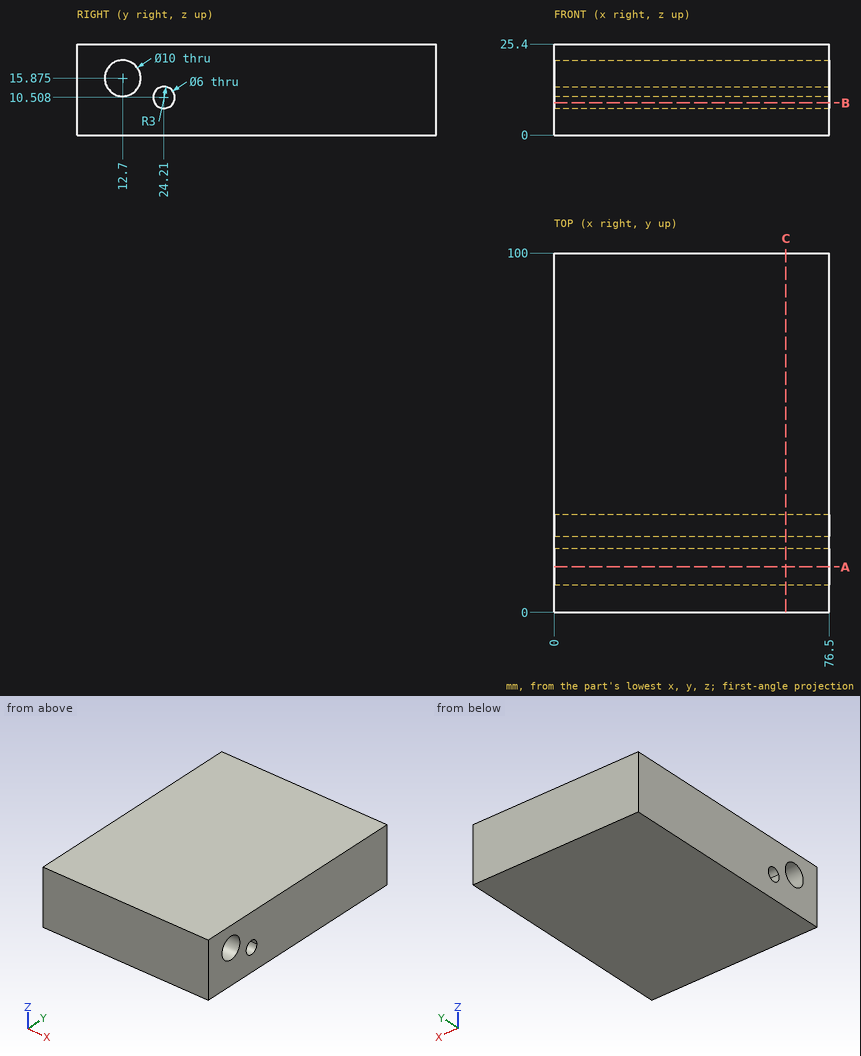
Design review of the part shown in the three views and the two pictorial views. Dimensions are in mm from the part's minimum x, y and z. Give positions to 0.01 mm unless a question says otherwise; leave off trailing zeros. Write each loop counter-clockwise with the first axis right and the second up, starting at its lowest first coordinate (ties: lowest second). Pieces come first, ordered by that corner, then holes.
Item 1: Insertion check: P1, Ø4, axis at x = 42, y = 51, coming from the -Z side. The pin has a flat end and moves straight along its axis. Give the tip position at first contact, or say it passes through.
Item 2: Take a section at C-C (x = 64.5). Give the boundary of the cut face in (y, z) (1 decimal), and give its area (3 significant figures).
Item 3: Take a section at A-A (y = 12.7). Give the boundary of the cut face in (x, z) (1 decimal).
Item 4: Wall thickness on probe 1 along Y at (x, z) = (27, 15.5); probe 2 along Y at (x, z) = (11.5, 12.25) (1 decimal); probe 3 along Y at (x, z) = (36, 12.75): over which ranges is each line inside the solid? List them lowest first.
Item 5: Take a section at B-B (z = 9). Give the boundary of the cut face in (x, y).
Established:
1. P1: stops at z = 0
2. outline: (0, 0) - (100, 0) - (100, 25.4) - (0, 25.4) - close; hole circle Ø10 at (12.7, 15.9); hole circle Ø6 at (24.2, 10.5)
2. area: 2,430 mm2
3. outline: (0, 0) - (76.5, 0) - (76.5, 10.9) - (0, 10.9) - close; (0, 20.9) - (76.5, 20.9) - (76.5, 25.4) - (0, 25.4) - close
4. probe 1: y = 0 to 7.71, 17.69 to 100
4. probe 2: y = 0 to 9.3, 16.1 to 21.8, 26.7 to 100
4. probe 3: y = 0 to 8.8, 16.6 to 22.22, 26.2 to 100
5. outline: (0, 0) - (76.5, 0) - (76.5, 21.62) - (0, 21.62) - close; (0, 26.8) - (76.5, 26.8) - (76.5, 100) - (0, 100) - close
